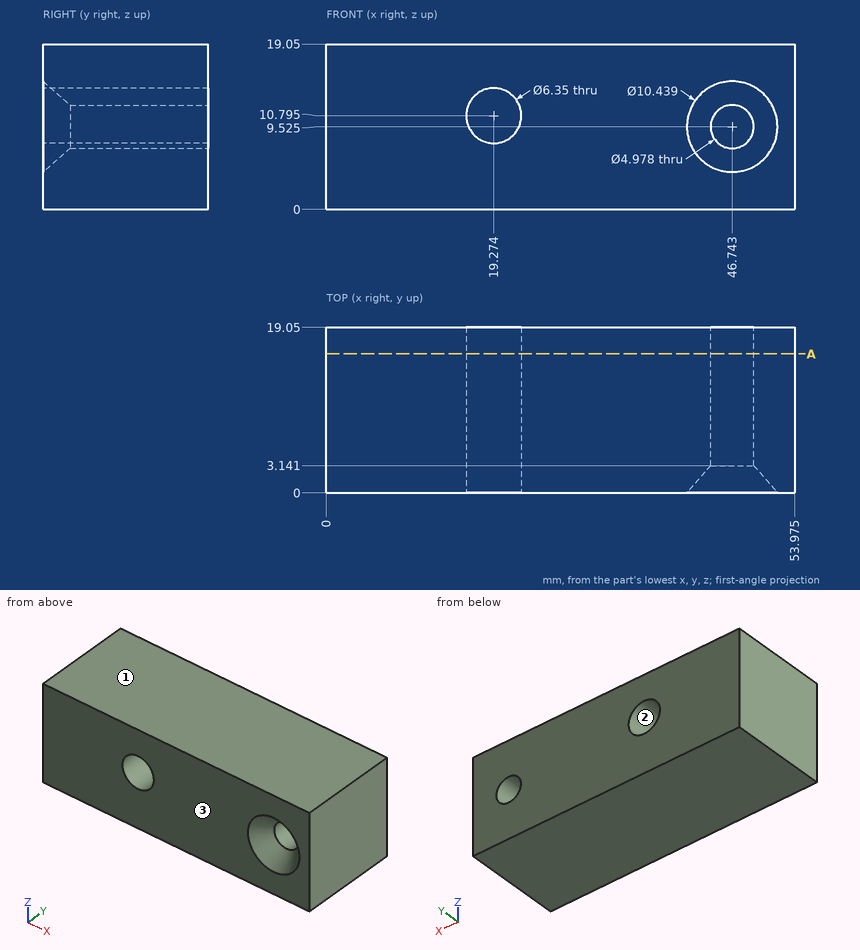
The drawing under review shows one solid part. Ordinate dimensions are in mm from its lowest x, y, z. Give positions to 0.01 mm unless a question says otherwise; leave off trailing zeros. Write item = value, one per line. Start each with the question number.
(1) We need section A-A on y = 16. State how many separate pieces and enclosed holes the cut face has, plus the area to 3 significant figures.
(2) To check wall thickness, follow line 1 along X through (y, z) = (10.75, 8) (1 decimal); line 2 along X through (y, z) = (12.25, 9) (1 decimal); line 3 along Z through (x, y) = (45, 14.25). State the ranges of each line that lie inside material, in increasing order.
(3) For pin 1 (5.5 mm diameter, centred on x = 19.27, z = 10.8, fed in from +Y), flat-tipped, find the tip position at first contact; note if it passes through.
(4) Mouldability with a two-part tool opening along Z and no side actions: class the marked faces 1, 2 and 3 as +Z half, -Z half, draft (parallel to the pull), parting line (faces both ways), or undercut.
Numbers:
q1.separate_pieces = 1
q1.enclosed_holes = 2
q1.area = 977 mm^2
q2.line_1 = 0 to 17.8, 20.8 to 44.8, 48.7 to 54
q2.line_2 = 0 to 16.7, 21.9 to 44.3, 49.2 to 54
q2.line_3 = 0 to 7.75, 11.3 to 19.05
q3.pin_1 = through
q4.face_1 = +Z half
q4.face_2 = undercut
q4.face_3 = draft
